Part model, mm, in its own coordinate system. A direction names the side the tool comes from. Give positions to 0.01 mm unless a question says otherwise; leave off trailing zeros. Order: outer loops, then holes, each group sorted by start corner. A loop starts at its lowest first (then second) coordinate and runs counter-clockwise, first axis right, second up. Notation, with made-up numbers: (80, 86.5) - (135, 86.5) arc R13 cw to (135, 102.5) - close; hole circle Ø2 at (-26, 23). An arc over 180 degrees is marked (long way). One line per item, written item: value.
```python
from build123d import *

# Parameters (mm, degrees)
EXTRUDE_1_DEPTH          = 10
EXTRUDE_1_DEPTH_BACK     = 10
EXTRUDE_2_DEPTH          = 10
EXTRUDE_2_DEPTH_BACK     = 10
CUT_EXTRUDE_1_DEPTH      = 78.86350451
CUT_EXTRUDE_2_DEPTH      = 331.104586341
CUT_EXTRUDE_2_DEPTH_BACK = 331.104586341
SKETCH_7_W               = 31.119179355
SKETCH_7_H               = 7.69001946
EXTRUDE_3_DEPTH          = 15
CUT_EXTRUDE_3_DEPTH      = 331.22914457
CUT_EXTRUDE_3_DEPTH_BACK = 331.22914457
CUT_EXTRUDE_4_DEPTH      = 3.5
CUT_EXTRUDE_5_DEPTH      = 5.121010883


with BuildPart() as part:
    # 草图3 → 凸台-拉伸1 (new, two sides: drawn at the far end of the back side and taken through both)
    with BuildSketch(Plane(origin=(0, 0, 0), x_dir=(1, 0, 0), z_dir=(0, 1, 0)).offset(-EXTRUDE_1_DEPTH_BACK)):
        Polygon((213.340896476, 89.860350871), (216.879610096, 89.860350871), (218.224577979, 95.937014496), (254.949012169, 95.937014496), (273.762340852, 180.937014496), (233.499193043, 180.937014496), align=None)
    extrude(amount=EXTRUDE_1_DEPTH + EXTRUDE_1_DEPTH_BACK)

    # 草图5 → 凸台-拉伸2 (add, two sides: drawn at the far end of the back side and taken through both)
    with BuildSketch(Plane(origin=(0, 0, 0), x_dir=(1, 0, 0), z_dir=(0, 1, 0)).offset(-EXTRUDE_2_DEPTH_BACK)):
        Polygon((271.991674623, 172.937014496), (275.918166689, 172.937014496), (258.875504234, 95.937014496), (254.949012169, 95.937014496), align=None)
    extrude(amount=EXTRUDE_2_DEPTH + EXTRUDE_2_DEPTH_BACK)

    # 草图6 → 切除-拉伸1 (cut, along a direction that is not the sketch's normal)
    with BuildSketch(Plane(origin=(0, 0, -172.937014496), x_dir=(-1, 0, 0), z_dir=(0, 0, -1))):
        Polygon((-275.918166689, 7), (-271.991674623, 9), (-271.991674623, 10), (-275.918166689, 10), align=None)
        Polygon((-271.991674623, -9), (-271.991674623, -10), (-275.918166689, -10), (-275.918166689, -7), align=None)
    extrude(amount=-CUT_EXTRUDE_1_DEPTH, dir=(0.21610328580589588, 0, -0.9763705084976171), mode=Mode.SUBTRACT)

    # 草图7 → 切除-拉伸2 (cut, two sides: drawn at the far end of the back side and taken through both)
    with BuildSketch(Plane(origin=(0, 0, 0), x_dir=(1, 0, 0), z_dir=(0, 1, 0)).offset(-CUT_EXTRUDE_2_DEPTH_BACK)):
        with Locations((213.489275448, 87.122004766)):
            Rectangle(SKETCH_7_W, SKETCH_7_H)
    extrude(amount=CUT_EXTRUDE_2_DEPTH + CUT_EXTRUDE_2_DEPTH_BACK, mode=Mode.SUBTRACT)

    # 草图8 → 凸台-拉伸3 (add)
    with BuildSketch(Plane.XY.offset(-95.937014496)):
        with BuildLine():
            Line((253.875504234, 13.5), (221.375504234, 13.5))
            ThreePointArc((221.375504234, 13.5), (214.304436422, 10.571067812), (211.375504234, 3.5))
            Line((211.375504234, 3.5), (211.375504234, -3.5))
            ThreePointArc((211.375504234, -3.5), (214.304436422, -10.571067812), (221.375504234, -13.5))
            Line((221.375504234, -13.5), (253.875504234, -13.5))
            ThreePointArc((253.875504234, -13.5), (260.946572046, -10.571067812), (263.875504234, -3.5))
            Line((263.875504234, -3.5), (263.875504234, 3.5))
            ThreePointArc((263.875504234, 3.5), (260.946572046, 10.571067812), (253.875504234, 13.5))
        make_face()
    extrude(amount=EXTRUDE_3_DEPTH)

    # 草图11 → 切除-拉伸3 (cut, two sides: drawn at the far end of the back side and taken through both)
    with BuildSketch(Plane(origin=(0, 0, 0), x_dir=(1, 0, 0), z_dir=(0, 1, 0)).offset(-CUT_EXTRUDE_3_DEPTH_BACK)):
        Polygon((268.062661222, 88.884668272), (201.658116102, 88.000919674), (201.658116102, 68.770636621), (268.062661222, 68.770636621), align=None)
    extrude(amount=CUT_EXTRUDE_3_DEPTH + CUT_EXTRUDE_3_DEPTH_BACK, mode=Mode.SUBTRACT)

    # 草图13 → 切除-拉伸4 (cut)
    with BuildSketch(Plane(origin=(0, 13.5, 0), x_dir=(1, 0, 0), z_dir=(0, 1, 0))):
        with BuildLine():
            Line((208, 90.937014496), (230.757405295, 90.937014496))
            ThreePointArc((230.757405295, 90.937014496), (234.708074056, 92.346011488), (236.875504234, 95.937014496))
            Line((236.875504234, 95.937014496), (236.875504234, 103.30474676))
            Line((236.875504234, 103.30474676), (208, 103.30474676))
            Line((208, 103.30474676), (208, 90.937014496))
        make_face()
    cut_extrude_4 = extrude(amount=-CUT_EXTRUDE_4_DEPTH, mode=Mode.SUBTRACT)

    # 镜向1: 切除-拉伸4 across plane
    add(cut_extrude_4.mirror(Plane.ZX), mode=Mode.SUBTRACT)

    # 草图14 → 切除-拉伸5 (cut, along a direction that is not the sketch's normal)
    with BuildSketch(Plane(origin=(0, 0, -95.937014496), x_dir=(-1, 0, 0), z_dir=(0, 0, -1))):
        with BuildLine():
            Line((-213.776162157, -10), (-214.68586436, -10))
            Line((-214.68586436, -10), (-214.68586436, 10))
            Line((-214.68586436, 10), (-213.776162157, 10))
            ThreePointArc((-213.776162157, 10), (-211.994848053, 6.964576398), (-211.375504234, 3.5))
            Line((-211.375504234, 3.5), (-211.375504234, -3.5))
            ThreePointArc((-211.375504234, -3.5), (-211.994848053, -6.964576398), (-213.776162157, -10))
        make_face()
    extrude(amount=-CUT_EXTRUDE_5_DEPTH, dir=(0.2161032858058959, 0, -0.9763705084976171), mode=Mode.SUBTRACT)


solid = part.part
```
1) Cut at D-D, the plane x = 235.5. Give the cut face in (y, z), then the cut area to 3 significant figures.
Outcome:
outline: (-13.5, -93.12) - (-10, -93.12) - (-10, -180.94) - (10, -180.94) - (10, -93.12) - (13.5, -93.12) - (13.5, -88.45) - (-13.5, -88.45) - close
area: 1,880 mm^2
2) Pin check, flat tips, straight feed: pin 1 (3 mm diameter, centred on x = 220.5, y = -12, fed in from -Z); pin 2 (4 mm diameter, centred on x = 261.5, z = -114, fed in from -Y); pin 3 (2 mm diameter, centred on y = -8.5, z = -104.5, fed in from -X). Stop position of each tip, or through.
Outcome:
pin 1: stops at z = -90.94
pin 2: stops at y = -8.74
pin 3: stops at x = 216.36
3) Drill centre lines: line 1 along Y through (x, z) = (219.5, -111); line 2 along Z through (x, y) = (255, 3.25); line 3 along Y through (x, z) = (262, -126.5). Where is each one in solid material? Low to high. Write a range as from..to.
Outcome:
line 1: y = -10..10
line 2: z = -180.94..-88.71
line 3: y = -8.85..8.85
4) Which spindle directions (+Z, -Z, +X, -X, +Y, -Y) get a long thin tool onto all of the face, cutting with end or side? Do faces 1 (the cylindrical face through (234.662, -11.774, -92.308)), 2 (the flat face through (212, 0, -90.937)), 3 (the cylindrical face through (261.024, 10.493, -92.367)), 4 (the flat face through (259.2, 0.2, -95.937)). Say none if no direction does.
Outcome:
face 1: -Z, -X, -Y
face 2: -Z, -X, +Y, -Y
face 3: +Z, +X, +Y
face 4: +X
5) Mould opens along Z. For faces 5 (the flat face through (241, -13.5, -91)), 6 (the flat face through (266, -8, -137)), 7 (the flat face through (254, 0, -180.937)) say: released by +Z, released by -Z, zero draft, split by the parting line, or undercut.
Outcome:
face 5: zero draft
face 6: undercut
face 7: released by -Z
6) Cut at C-C, the plane z = -116. Give the cut face in (x, y).
Outcome:
outline: (219.13, -10) - (259.39, -10) - (259.39, -9) - (263.32, -7) - (263.32, 7) - (259.39, 9) - (259.39, 10) - (219.13, 10) - close
7) Cut at B-B, the plane y = 1. Give the cut face in (x, z), then the cut area to 3 significant figures.
Outcome:
outline: (211.38, -90.94) - (213.58, -90.94) - (233.5, -180.94) - (273.76, -180.94) - (271.99, -172.94) - (275.92, -172.94) - (258.88, -95.94) - (263.88, -95.94) - (263.88, -88.83) - (211.38, -88.13) - close
area: 4,100 mm^2
8) Cut at A-A, the plane x = 261. Give the cut face in (y, z).
Outcome:
outline: (-10.52, -95.94) - (10.52, -95.94) - (10.52, -88.79) - (-10.52, -88.79) - close; (-10, -180.94) - (10, -180.94) - (10, -123.28) - (9, -123.28) - (7, -105.54) - (-7, -105.54) - (-9, -123.28) - (-10, -123.28) - close
